```python
from build123d import *

# Parameters (mm, degrees)
SKETCH_1_W          = 100
SKETCH_1_H          = 20
EXTRUDE_1_DEPTH     = 3
FILLET_1_R          = 10
SKETCH_4_W          = 20
SKETCH_4_H          = 3
EXTRUDE_2_DEPTH     = 20
FILLET_2_R          = 10
SKETCH_5_R          = 5
CUT_EXTRUDE_1_DEPTH = 10
SKETCH_5_3_R        = 5
CUT_EXTRUDE_2_DEPTH = 10


with BuildPart() as part:
    # ｽｹｯﾁ1 → ﾎﾞｽ - 押し出し1 (new body)
    with BuildSketch(Plane.XY):
        with Locations((50, 10)):
            Rectangle(SKETCH_1_W, SKETCH_1_H)
    extrude(amount=EXTRUDE_1_DEPTH)

    # ﾌｨﾚｯﾄ1
    fillet_1_edges = [part.edges().sort_by_distance(p)[0] for p in [
        (100, 0, 1.5),
        (100, 20, 1.5),
        (0, 0, 1.5),
        (0, 20, 1.5),
    ]]
    fillet(fillet_1_edges, radius=FILLET_1_R - 0.0001)  # a hair under: the kernel refuses the full size

    # ｽｹｯﾁ4 → ﾎﾞｽ - 押し出し2 (add)
    with BuildSketch(Plane(origin=(0, 20, 0), x_dir=(1, 0, 0), z_dir=(0, 1, 0))):
        with Locations((50, -1.5)):
            Rectangle(SKETCH_4_W, SKETCH_4_H)
    extrude(amount=EXTRUDE_2_DEPTH)

    # ﾌｨﾚｯﾄ2
    fillet_2_edges = [part.edges().sort_by_distance(p)[0] for p in [
        (40, 40, 1.5),
        (60, 40, 1.5),
    ]]
    fillet(fillet_2_edges, radius=FILLET_2_R - 0.0001)  # a hair under: the kernel refuses the full size

    # ｽｹｯﾁ5 → ｶｯﾄ - 押し出し1 (cut)
    with BuildSketch(Plane.XY.offset(3)):
        with Locations((10, 10)):
            Circle(SKETCH_5_R)
    extrude(amount=-CUT_EXTRUDE_1_DEPTH, mode=Mode.SUBTRACT)

    # ｽｹｯﾁ5<3> → ｶｯﾄ - 押し出し2 (cut)
    with BuildSketch(Plane.XY.offset(3)):
        with Locations((50, 29.784394475)):
            Circle(SKETCH_5_3_R)
        with Locations((10, 10)):
            Circle(SKETCH_5_3_R)
        with Locations((90, 10)):
            Circle(SKETCH_5_3_R)
    extrude(amount=-CUT_EXTRUDE_2_DEPTH, mode=Mode.SUBTRACT)


solid = part.part
```
Can you work these out from the model? Positions are in its coordinate system, mm. A direction names the side the tool comes from. Round coordinates to 2 decimals unless told otherwise and drop trailing zeros. Loops run counter-clockwise (first coordinate to the right, second up) from the corner with the lowest first, then second, coordinate; pieces in that order, holes last. Notation, with made-up numbers: (-2.75, -40) -> (5.25, -40) arc R19 cw to (5.25, -15) -> close; hole circle Ø9 at (25.25, -33.75). An arc over 180 degrees is marked (long way). Answer in a Markdown table with one row per item.
Item 1: We'd pull the mould along Y, two halves only. Please class faces 4 (the flat face through (49, 0, 1)), 5 (the cylindrical face through (94.619, 8.085, 1.521)), 6 (the cylindrical face through (14.77, 11.5, 1.52)), 7 (the flat face through (40, 25, 2)): released by +Y, released by -Y, zero draft, split by the parting line, or undercut.
Answer block:
| item | result |
|---|---|
| face 4 | released by -Y |
| face 5 | undercut |
| face 6 | undercut |
| face 7 | zero draft |
Item 2: Suppose I cut it at C-C, the plane x = 69. List the corners of the cut face in (y, z) for me, plus the area to 3 significant figures.
Answer block:
| item | result |
|---|---|
| outline | (0, 0) -> (20, 0) -> (20, 3) -> (0, 3) -> close |
| area | 60.0 mm² |
Item 3: Suppose I cut it at B-B, the plane z = 1.8. Give the number of separate pieces and of enclosed holes in the cut face, plus the area to 3 significant figures.
Answer block:
| item | result |
|---|---|
| separate pieces | 1 |
| enclosed holes | 3 |
| area | 2,040 mm² |
Item 4: On a 3-axis mill with a long thin cutter (end or side, diameter ignored), from which of +Z, -Z, +X, -X, +Y, -Y can I reach the whole of each face in a straight line? I mean faces 1 (the flat face through (75, 20, 1)), 2 (the flat face through (25, 20, 1)), 3 (the cylindrical face through (48.916, 24.903, 1.521)). Say none if no direction works.
Answer block:
| item | result |
|---|---|
| face 1 | +Z, -Z, +X, +Y |
| face 2 | +Z, -Z, -X, +Y |
| face 3 | +Z, -Z |
Item 5: Suppose I cut it at D-D, the plane y = 23. List the corners of the cut face in (x, z) for me.
Answer block:
| item | result |
|---|---|
| outline | (40, 0) -> (60, 0) -> (60, 3) -> (40, 3) -> close |
Item 6: Suppose I cut it at A-A, the plane y = 14. List the corners of the cut face in (x, z) for me, plus the area to 3 significant figures.
Answer block:
| item | result |
|---|---|
| outline | (0.83, 0) -> (7, 0) -> (7, 3) -> (0.83, 3) -> close; (13, 0) -> (87, 0) -> (87, 3) -> (13, 3) -> close; (93, 0) -> (99.17, 0) -> (99.17, 3) -> (93, 3) -> close |
| area | 259 mm² |
Item 7: If I drill on probe 1 along Y at (x, z) = (50, 0.8); probe 2 along Y at (x, z) = (10, 1); probe 3 along X at (y, z) = (11.5, 0.9), over which ranges is the centre line in solid material (lowest first)?
Answer block:
| item | result |
|---|---|
| probe 1 | 0 to 24.78, 34.78 to 40 |
| probe 2 | 0 to 5, 15 to 20 |
| probe 3 | 0.11 to 5.23, 14.77 to 85.23, 94.77 to 99.89 |
Item 8: Will these pins go through, and if not, where does the flat tip stop? P1, Ø0.9, axis at y = 25.5, z = 1.5, coming from the -X side; P2, Ø0.9, axis at x = 78, z = 2, coming from the +Y side; P3, Ø1.5, axis at y = 24.5, z = 1, coming from the +X side.
Answer block:
| item | result |
|---|---|
| P1 | x = 40 |
| P2 | y = 20 |
| P3 | x = 60 |
